```python
from build123d import *

# Parameters (mm, degrees)
SKETCH1_R           = 12.7
BOSS_EXTRUDE1_DEPTH = 39.751
SKETCH2_R           = 8.73125
CUT_EXTRUDE1_DEPTH  = 30.226
SKETCH4_R           = 7.62
BOSS_EXTRUDE2_DEPTH = 6.35
SKETCH5_R           = 3.175
BOSS_EXTRUDE3_DEPTH = 1.5875
SKETCH7_R           = 12.7
BOSS_EXTRUDE4_DEPTH = 12.7
CHAMFER1_SIZE       = 1.524


# Read off the part's stored shape, not the designer's step: 1/8 NPT Tapped Hole1
with BuildPart() as part:
    # Sketch1 → Boss-Extrude1 (new body)
    with BuildSketch(Plane(origin=(0, 0, 0), x_dir=(1, 0, 0), z_dir=(0, 1, 0))):
        with Locations(Location((0, 0, 0), (0, 0, 270))):
            Circle(SKETCH1_R)
    extrude(amount=BOSS_EXTRUDE1_DEPTH)

    # Sketch2 → Cut-Extrude1 (cut)
    with BuildSketch(Plane.XZ):
        with Locations(Location((0, 0, 0), (0, 0, 270))):
            Circle(SKETCH2_R)
    extrude(amount=-CUT_EXTRUDE1_DEPTH, mode=Mode.SUBTRACT)

    # Sketch4 → Boss-Extrude2 (add)
    with BuildSketch(Plane(origin=(0, 39.751, 0), x_dir=(1, 0, 0), z_dir=(0, 1, 0))):
        with Locations(Location((0, 0, 0), (0, 0, 270))):
            Circle(SKETCH4_R)
    extrude(amount=BOSS_EXTRUDE2_DEPTH)

    # Sketch5 → Boss-Extrude3 (add)
    with BuildSketch(Plane(origin=(0, 46.101, 0), x_dir=(1, 0, 0), z_dir=(0, 1, 0))):
        with Locations(Location((0, 0, 0), (0, 0, 270))):
            Circle(SKETCH5_R)
    extrude(amount=BOSS_EXTRUDE3_DEPTH)

    # Sketch7 → Boss-Extrude4 (add)
    with BuildSketch(Plane(origin=(0, 47.6885, 0), x_dir=(1, 0, 0), z_dir=(0, 1, 0))):
        with Locations(Location((0, 0, 0), (0, 0, 270))):
            Circle(SKETCH7_R)
    extrude(amount=BOSS_EXTRUDE4_DEPTH)

    # Chamfer1
    chamfer1_edges = [part.edges().sort_by_distance(p)[0] for p in [
        (0, 47.6885, -12.7),
        (0, 60.3885, -12.7),
        (0, 39.751, -12.7),
    ]]
    chamfer(chamfer1_edges, length=CHAMFER1_SIZE)

    # 1/8 NPT Tapped Hole1 outline → 1/8 NPT Tapped Hole1 (revolve, cut)
    with BuildSketch(Plane.XZ.offset(-21.59)):
        Polygon((5.141518805, 12.700000181), (0, 12.700000181), (0, 7.174156466), (4.976067645, 7.174156466), align=None)
    revolve(axis=Axis((0, 21.59, 0), (0, 0, 1)), mode=Mode.SUBTRACT)


solid = part.part
```
Check sheet for the modelled part. Datum: model origin and axes. Units: mm. A direction names the side the tool comes from. Coordinates: 2 decimals unless noted, no trailing zeros. Order: outer loops, then holes, each group sorted by start corner. A loop starts at its lowest first (then second) coordinate and runs counter-clockwise, first axis right, second up. Notation, with made-up numbers: (78.5, 89) -> (96.5, 89) arc R27 ccw to (96.5, 112) -> close; hole circle Ø5 at (50, 31.25). An arc over 180 degrees is marked (long way). Write item = value, one per line. Start each with the question number.
1) Mould release check, pull along Z, two halves, no side actions. Record for faces 1 (the cylindrical face through (2.62, 14.9, -8.33)), 2 (the cylindrical face through (7.555, 42.882, -0.992)), 3 (the conical face through (-4.015, 18.511, 9.976)): +Z half, -Z half, draft (parallel to the pull), parting line (faces both ways), or undercut.
2) Cross-section at D-D (y = 21.59). Enter the section's corners in (x, z), then the cut area to 3 significant figures.
3) Material ranges on L1, parallel to Y at x = -2.5, z = -6.25; L2, parallel to Y at x = 7, z = -8.5; L3, parallel to X at y = 19.5, z = 0, recorded low to high.
4) Cross-section at C-C (y = 43). Enter the section's corners in (x, z), then the cut area to 3 significant figures.
5) Cross-section at A-A (z = 0). Enter the section's corners in (x, y) (1 decimal).
6) Go/stop test with flat-tipped pins: P1, Ø4, axis at x = 6, y = 27.5, coming from the -Z side; P2, Ø2, axis at y = 9.5, z = -2.5, coming from the +X side; P3, Ø5, axis at x = 4.5, y = 6, coming from the -Z side. Record where each tip stops, or that it passes through.
7) Access from +Z, -Z, +X, -X, +Y, -Y to the whole of each face (thin tool, end or side, straight path). Record for faces 4 (the flat face through (-7, 39.751, 5)), 5 (the flat face through (0, 60.388, 0)), 6 (the flat face through (0, 30.226, 0)).
Ans:
q1.face_1 = undercut
q1.face_2 = parting line
q1.face_3 = +Z half
q2.outline = (-5.11, 11.63) arc R12.7 ccw (long way) to (5.11, 11.63) -> (4.98, 7.17) arc R8.73 cw (long way) to (-4.98, 7.17) -> close
q2.area = 225 mm²
q3.L1 = 30.23 to 46.1, 47.69 to 60.39
q3.L2 = 0 to 39.75, 47.69 to 60.39
q3.L3 = -12.7 to -8.73, 8.73 to 12.7
q4.outline = circle Ø15.24 at (0, 0)
q4.area = 182 mm²
q5.outline = (-12.7, 0) -> (-8.7, 0) -> (-8.7, 30.2) -> (8.7, 30.2) -> (8.7, 0) -> (12.7, 0) -> (12.7, 38.2) -> (11.2, 39.8) -> (7.6, 39.8) -> (7.6, 46.1) -> (3.2, 46.1) -> (3.2, 47.7) -> (11.2, 47.7) -> (12.7, 49.2) -> (12.7, 58.9) -> (11.2, 60.4) -> (-11.2, 60.4) -> (-12.7, 58.9) -> (-12.7, 49.2) -> (-11.2, 47.7) -> (-3.2, 47.7) -> (-3.2, 46.1) -> (-7.6, 46.1) -> (-7.6, 39.8) -> (-11.2, 39.8) -> (-12.7, 38.2) -> close
q6.P1 = -12.05
q6.P2 = 12.61
q6.P3 = -12.54
q7.face_4 = none
q7.face_5 = +Z, -Z, +X, -X, +Y
q7.face_6 = -Y
